Part model, mm, in its own coordinate system. Give positions to 0.01 mm unless a question says otherwise; leave off trailing zeros. Write each loop counter-clockwise with the first axis right and the second up, starting at its lowest first coordinate (ties: lowest second). Pieces come first, ordered by that corner, then holes. Notation, with made-up numbers: M -11.5,-31 L 4.5,-31 A18 cw 4.5,0 Z; hole C -11,-40 d11. An arc over 180 degrees is marked long. Write item = value, one per line. Start each with the question number.
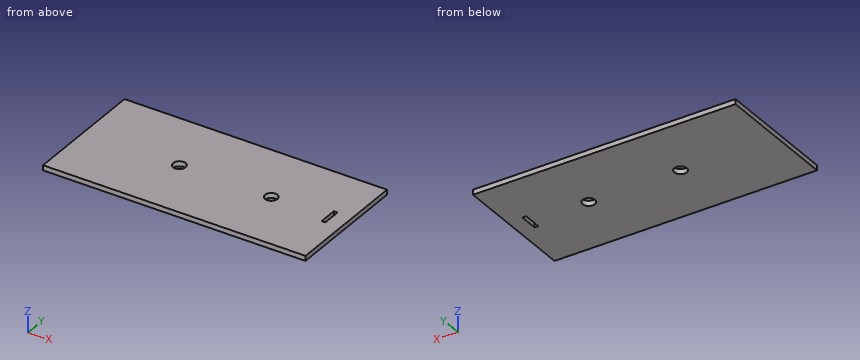
from build123d import *

# Parameters (mm, degrees)
SKETCH1_W           = 210
SKETCH1_H           = 100
SKETCH1_R           = 5
SKETCH1_W_2         = 3
SKETCH1_H_2         = 15
BOSS_EXTRUDE1_DEPTH = 4


with BuildPart() as part:
    # Sketch1 → Boss-Extrude1 (new body)
    with BuildSketch(Plane.XY):
        with Locations((-45, 0)):
            Rectangle(SKETCH1_W, SKETCH1_H)
        Circle(SKETCH1_R, mode=Mode.SUBTRACT)
        with Locations((-73.5, 0)):
            Circle(SKETCH1_R, mode=Mode.SUBTRACT)
        with Locations((46.5, 0.26206532)):
            Rectangle(SKETCH1_W_2, SKETCH1_H_2, mode=Mode.SUBTRACT)
    extrude(amount=BOSS_EXTRUDE1_DEPTH)


solid = part.part
Q1. Slice it at A-A (x = -73.5). Give the cut face in (y, z).
Q2. Probe line 1 along Y through (x, z) = (0, 0.95); line 2 along X through (y, z) = (3, 3.85); line 3 along Y through (x, z) = (-3, 2.7). List the from-to ranges inside material, lowest first.
Q3. Slice it at B-B (y = 0). Give the cut face in (x, z).
Working result:
q1.outline = M -50,0 L -5,0 L -5,4 L -50,4 Z; M 5,0 L 50,0 L 50,4 L 5,4 Z
q2.line_1 = -50 to -5, 5 to 50
q2.line_2 = -150 to -77.5, -69.5 to -4, 4 to 45, 48 to 60
q2.line_3 = -50 to -4, 4 to 50
q3.outline = M -150,0 L -78.5,0 L -78.5,4 L -150,4 Z; M -68.5,0 L -5,0 L -5,4 L -68.5,4 Z; M 5,0 L 45,0 L 45,4 L 5,4 Z; M 48,0 L 60,0 L 60,4 L 48,4 Z
